The listing builds one solid part. Answer for the finished solid, in the listing's coordinates (mm). Face numbers are marked on the shaded views. A direction names the side the tool comes from. Coordinates: 2 decimals unless noted, no trailing zeros. Loops run counter-clockwise (first coordinate to the right, second up) from the corner with the lowest first, then second, coordinate; pieces in that order, holes last. Notation, with made-up numbers: (20, 67) - (78, 67) arc R16 ccw to (78, 98) - close; hole circle Ø4 at (59.5, 6.25). An arc over 180 degrees is marked (long way). Return JSON: item names as keys, results as strings. Group by question number.
1. The mould has two halves that part along X. Classify the marked faces 4, 5 and 6: pulls with the +X half, pulls with the -X half, needs draft (parallel to the pull), parting line crosses it, or undercut.
2. Section D-D (x = 6.5) is taken. Write down the section's boundary in (y, z) (3 decimals), and give its area (3 significant figures).
3. Find the intervals of material crossed by line 1 along Z through (x, y) = (-27.5, 2.5) (3 decimals); line 2 along Z through (x, y) = (-31.5, -2); line 3 along Z through (x, y) = (-21.7, -5) (3 decimals), in increasing order.
4. Which of the six approach directions +Z, -Z, +X, -X, +Y, -Y give full straight-line access (tool end or side, diameter ignored) to the marked faces 1, 2 and 3?
5. Section B-B (y = -12.25) is taken. Write down the section's boundary in (x, z), and give its area (3 significant figures).
6. Section A-A (y = -6.25) is taken. State how many separate pieces and enclosed holes the cut face has, and give its area (3 significant figures).
7. Each of these flat-tipped pins is pushed along its axis until it touches: P1, Ø5, axis at y = -7, z = -18.5, coming from the +X side (3 decimals); P2, Ø1.6, axis at y = -6, z = -1, coming from the +X side; P3, Ø2, axis at x = -3.5, y = -0.5, coming from the -Z side; P4, Ø8, axis at x = -30.5, y = 5, coming from the -Z side. Where does it stop, or does it pass through?
8. Section C-C (z = -17.5) is taken. Write down the section's boundary in (x, y) (3 decimals), and give its area (3 significant figures).
```python
from build123d import *

# Parameters (mm, degrees)
BOSS_EXTRUDE1_DEPTH                              = 7.5
SKETCH6_W                                        = 19
SKETCH6_H                                        = 15
SKETCH6_W_2                                      = 15
SKETCH6_H_2                                      = 11
BOSS_EXTRUDE3_DEPTH                              = 15
M3_CLEARANCE_HOLE1_D                             = 3.25
CBORE_FOR_M5_HEX_HEAD_MACHINE_SCREW1_D           = 4.25
CBORE_FOR_M5_HEX_HEAD_MACHINE_SCREW1_CBORE_D     = 5
CBORE_FOR_M5_HEX_HEAD_MACHINE_SCREW1_CBORE_DEPTH = 0.5
SKETCH3_R                                        = 8.75
SKETCH3_R_2                                      = 5.125
BOSS_EXTRUDE4_DEPTH                              = 10
CBORE_FOR_M3_SHCS1_D                             = 4.25
CBORE_FOR_M3_SHCS1_DEPTH                         = 10
CBORE_FOR_M3_SHCS1_CBORE_D                       = 5.25
CBORE_FOR_M3_SHCS1_CBORE_DEPTH                   = 0.5
CBORE_FOR_M3_SHCS2_D                             = 4.25
CBORE_FOR_M3_SHCS2_DEPTH                         = 10
CBORE_FOR_M3_SHCS2_CBORE_D                       = 5.25
CBORE_FOR_M3_SHCS2_CBORE_DEPTH                   = 0.5
CUT_EXTRUDE1_START                               = -5
SKETCH15_R                                       = 5.125
CUT_EXTRUDE1_DEPTH                               = 5


with BuildPart() as part:
    # Sketch1 → Boss-Extrude1 (new body)
    with BuildSketch(Plane(origin=(0, 0, 0), x_dir=(1, 0, 0), z_dir=(0, 1, 0))):
        with BuildLine():
            Line((-38.125, 18.75), (-38.125, -18.75))
            ThreePointArc((-38.125, -18.75), (-32.843579255, -27.566745988), (-22.577998038, -27.070502943))
            Line((-22.577998038, -27.070502943), (5.547001962, -8.320502943))
            ThreePointArc((5.547001962, -8.320502943), (10, 0), (5.547001962, 8.320502943))
            Line((5.547001962, 8.320502943), (-22.577998038, 27.070502943))
            ThreePointArc((-22.577998038, 27.070502943), (-32.843579255, 27.566745988), (-38.125, 18.75))
        make_face()
    extrude(amount=BOSS_EXTRUDE1_DEPTH)

    # Sketch6 → Boss-Extrude3 (add)
    with BuildSketch(Plane.XZ):
        with Locations((-27.5, 0)):
            Rectangle(SKETCH6_W, SKETCH6_H)
        with Locations((-27.5, 0)):
            Rectangle(SKETCH6_W_2, SKETCH6_H_2, mode=Mode.SUBTRACT)
    extrude(amount=BOSS_EXTRUDE3_DEPTH)

    # M3 Clearance Hole1 (through all)
    with Locations(Plane.XZ):
        with Locations((-27.5, 0)):
            Hole(M3_CLEARANCE_HOLE1_D / 2)

    # CBORE for M5 Hex Head Machine Screw1 (through all)
    with Locations(Plane(origin=(0, 7.5, 0), x_dir=(1, 0, 0), z_dir=(0, 1, 0))):
        with Locations((-12, 0)):
            CounterBoreHole(CBORE_FOR_M5_HEX_HEAD_MACHINE_SCREW1_D / 2, CBORE_FOR_M5_HEX_HEAD_MACHINE_SCREW1_CBORE_D / 2, CBORE_FOR_M5_HEX_HEAD_MACHINE_SCREW1_CBORE_DEPTH)

    # Sketch3 → Boss-Extrude4 (add)
    # profile 1 of 3: a face of its own
    with BuildSketch(Plane.XZ):
        with Locations(Location((-28.125, 18.75, 0), (0, 0, 90))):
            Circle(SKETCH3_R)
        with Locations(Location((-28.125, 18.75, 0), (0, 0, 270))):
            Circle(SKETCH3_R_2, mode=Mode.SUBTRACT)
    # profile 2 of 3: a face of its own
    with BuildSketch(Plane.XZ):
        with Locations(Location((-28.125, -18.75, 0), (0, 0, 90))):
            Circle(SKETCH3_R)
        with Locations(Location((-28.125, -18.75, 0), (0, 0, 270))):
            Circle(SKETCH3_R_2, mode=Mode.SUBTRACT)
    # profile 3 of 3: a face of its own
    with BuildSketch(Plane.XZ):
        with Locations(Location((0, 0, 0), (0, 0, 90))):
            Circle(SKETCH3_R)
        with Locations(Location((0, 0, 0), (0, 0, 270))):
            Circle(SKETCH3_R_2, mode=Mode.SUBTRACT)
    extrude(amount=BOSS_EXTRUDE4_DEPTH)

    # CBORE for M3 SHCS1
    with Locations(Plane(origin=(-19.375, 0, 0), x_dir=(0, 0, -1), z_dir=(1, 0, 0))):
        with Locations((-18.75, -5), (18.75, -5)):
            CounterBoreHole(CBORE_FOR_M3_SHCS1_D / 2, CBORE_FOR_M3_SHCS1_CBORE_D / 2, CBORE_FOR_M3_SHCS1_CBORE_DEPTH, depth=CBORE_FOR_M3_SHCS1_DEPTH)

    # CBORE for M3 SHCS2
    with Locations(Plane(origin=(8.75, 0, 0), x_dir=(0, 0, -1), z_dir=(1, 0, 0))):
        with Locations((0, -5)):
            CounterBoreHole(CBORE_FOR_M3_SHCS2_D / 2, CBORE_FOR_M3_SHCS2_CBORE_D / 2, CBORE_FOR_M3_SHCS2_CBORE_DEPTH, depth=CBORE_FOR_M3_SHCS2_DEPTH)

    # Sketch15 → Cut-Extrude1 (cut)
    with BuildSketch(Plane.XZ.offset(CUT_EXTRUDE1_START)):
        with Locations(Location((-28.125, 18.75, 0), (0, 0, 270))):
            Circle(SKETCH15_R)
        with Locations(Location((0, 0, 0), (0, 0, 270))):
            Circle(SKETCH15_R)
        with Locations(Location((-28.125, -18.75, 0), (0, 0, 270))):
            Circle(SKETCH15_R)
    extrude(amount=CUT_EXTRUDE1_DEPTH, mode=Mode.SUBTRACT)


solid = part.part
```
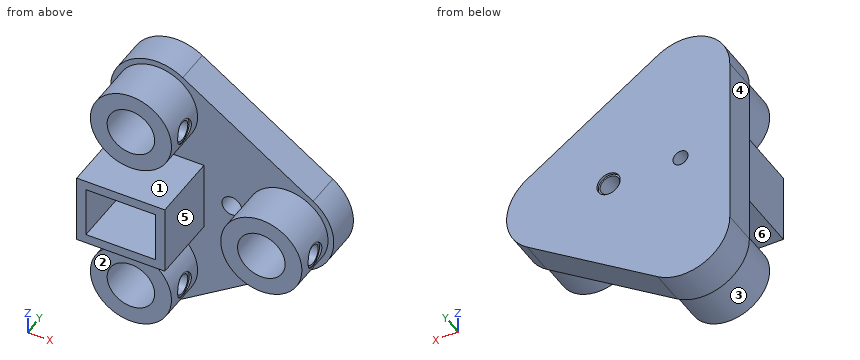
The answers:
{
 "1": {"face 4": "pulls with the -X half", "face 5": "undercut", "face 6": "needs draft"},
 "2": {"outline": "(-10, -5.858) - (0, -5.858) - (0, -7.599) - (7.5, -7.599) - (7.5, 7.599) - (0, 7.599) - (0, 5.858) - (-10, 5.858) - close; hole circle Ø4.25 at (-5, 0)", "area": "217 mm2"},
 "3": {"line 1": "z = -28.73 to -23.837, -13.663 to -1.625, 1.625 to 13.663, 23.837 to 28.73", "line 2": "z = -26.82 to -22.61, -14.89 to -10.68, -7.5 to -5.5, 5.5 to 7.5, 10.68 to 14.89, 22.61 to 26.82", "line 3": "z = -24.69 to -20.875, -16.625 to -12.81, -7.5 to -5.5, 5.5 to 7.5, 12.81 to 16.625, 20.875 to 24.69"},
 "4": {"face 1": "-X, -Y", "face 2": "-Z, +X, -X, -Y", "face 3": "-Y"},
 "5": {"outline": "(-37, -7.5) - (-18, -7.5) - (-18, 7.5) - (-37, 7.5) - close; hole (-35, -5.5) - (-20, -5.5) - (-20, 5.5) - (-35, 5.5) - close", "area": "120 mm2"},
 "6": {"separate pieces": "4", "enclosed holes": "1", "area": "555 mm2"},
 "7": {"P1": "stops at x = -19.375", "P2": "stops at x = 8.25", "P3": "stops at z = -14.93", "P4": "stops at z = -28.75"},
 "8": {"outline": "(-38.125, 0) - (-36.785, 0) - (-36.785, -10) - (-33.095, -10) - (-33.095, 5) - (-23.155, 5) - (-23.155, -3.282) - (-19.875, -3.282) - (-19.875, -2.692) - (-19.465, -2.692) - (-19.465, 0) - (-8.222, 0) - (-8.222, 7.5) - (-38.125, 7.5) - close; (-23.155, -10) - (-19.465, -10) - (-19.465, -7.308) - (-19.875, -7.308) - (-19.875, -6.718) - (-23.155, -6.718) - close", "area": "235 mm2"}
}
